Drawing for the job (mm, zero at the part's lowest x, y, z). A direction names the side the tool comes from. Round coordinates to 2 decimals unless told otherwise and drop trailing zeros. Write each loop counter-clockwise with the first axis right and the second up, starting at its lowest first coordinate (ties: lowest second). Pieces come first, ordered by that corner, then holes. Notation, with made-up numbers: (36, 35.25) - (90, 35.25) arc R16 cw to (90, 58.25) - close; hole circle Ø9 at (-13, -24). An arc over 180 degrees is marked (long way). Answer in a Markdown table with one row per item.
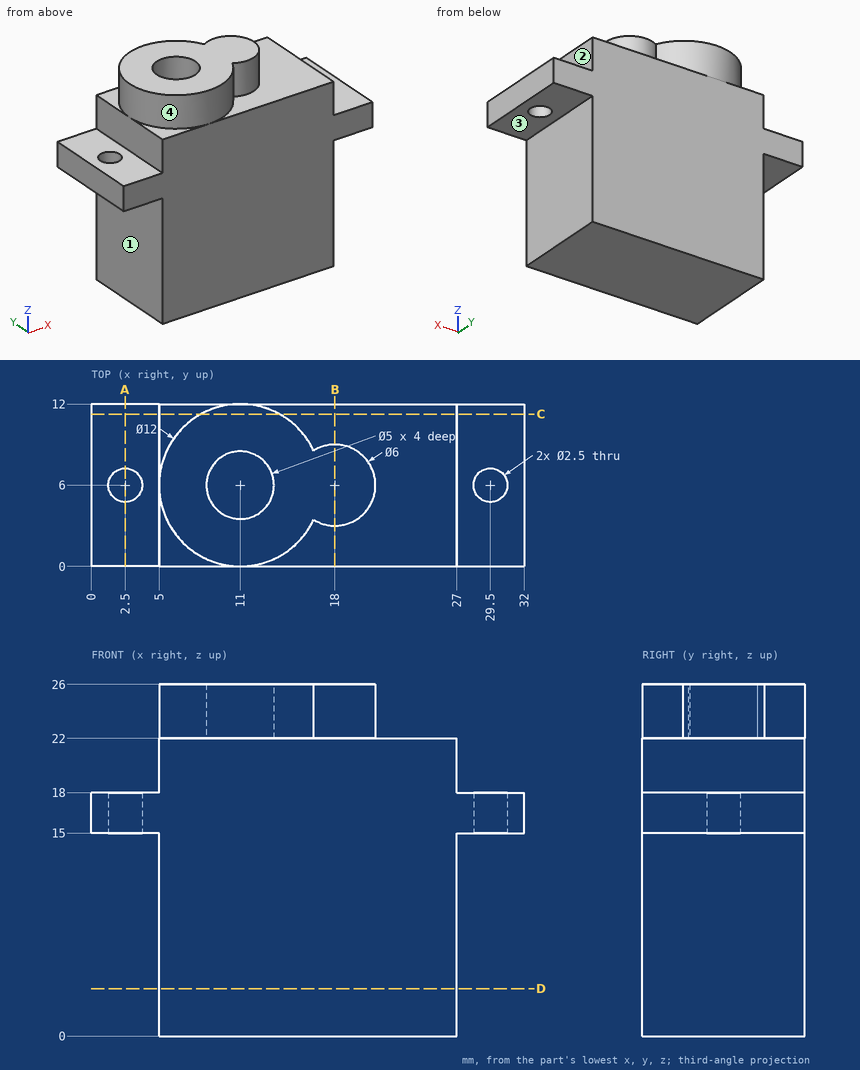
Q1. Saw through at D-D on z = 3.5. List the corners of the cut face in (x, y).
Computed:
| item | result |
|---|---|
| outline | (5, 0) - (27, 0) - (27, 12) - (5, 12) - close |
Q2. Flat gauge pins, fed straight in: pin 1 (3 mm diameter, centred on x = 24.5, y = 5.5, fed in from +Z); pin 2 (2.5 mm diameter, centred on x = 29, y = 8.5, fed in from -Z); pin 3 (2 mm diameter, centred on y = 2, z = 9, fed in from +X). Where does each tip first touch, or does it go through?
Computed:
| item | result |
|---|---|
| pin 1 | stops at z = 22 |
| pin 2 | stops at z = 15 |
| pin 3 | stops at x = 27 |
Q3. Saw through at C-C on y = 11.25. List the corners of the cut face in (x, z), then the cut area to 3 significant figures.
Computed:
| item | result |
|---|---|
| outline | (0, 15) - (5, 15) - (5, 0) - (27, 0) - (27, 15) - (32, 15) - (32, 18) - (27, 18) - (27, 22) - (13.9, 22) - (13.9, 26) - (8.1, 26) - (8.1, 22) - (5, 22) - (5, 18) - (0, 18) - close |
| area | 537 mm2 |
Q4. Saw through at B-B on x = 18. List the corners of the cut face in (y, z).
Computed:
| item | result |
|---|---|
| outline | (0, 0) - (12, 0) - (12, 22) - (9, 22) - (9, 26) - (3, 26) - (3, 22) - (0, 22) - close |
Q5. Drill centre lines: line 1 (Y direction, x = 29.5, z = 16.95); line 2 (Y direction, x = 11, z = 22.9); line 3 (X direction, y = 7, z = 15.5). Where is each one in solid material? Low to high.
Computed:
| item | result |
|---|---|
| line 1 | y = 0 to 4.75, 7.25 to 12 |
| line 2 | y = 0 to 3.5, 8.5 to 12 |
| line 3 | x = 0 to 1.75, 3.25 to 28.75, 30.25 to 32 |
Q6. 3-axis set-ups, long thin cutter, end or side, ignore diameter. For the marked faces 1, 2, 3 and 4: which of +Z, -Z, +X, -X, +Y, -Y reach the whole face in a straight line?
Computed:
| item | result |
|---|---|
| face 1 | -Z, -X, +Y, -Y |
| face 2 | +Z, +X, +Y, -Y |
| face 3 | -Z, +X, +Y, -Y |
| face 4 | +Z |
Q7. Saw through at A-A on x = 2.5. List the corners of the cut face in (y, z).
Computed:
| item | result |
|---|---|
| outline | (0, 15) - (4.75, 15) - (4.75, 18) - (0, 18) - close; (7.25, 15) - (12, 15) - (12, 18) - (7.25, 18) - close |
